from build123d import *


with BuildPart() as part:
    # Sketch1 → Revolve1 (revolve)
    with BuildSketch(Plane(origin=(0, 0, 0), x_dir=(0, 0, -1), z_dir=(1, 0, 0)), mode=Mode.PRIVATE) as revolve1_sk:
        with BuildLine():
            Line((-0.85, 1.95), (2.03, 1.95))
            Line((2.03, 1.95), (2.03, 1.5))
            Line((2.03, 1.5), (2.186173248, 1.2295))
            Line((2.186173248, 1.2295), (6.123826752, 1.2295))
            Line((6.123826752, 1.2295), (6.28, 1.5))
            Line((6.28, 1.5), (6.28, 2.100269256))
            Line((6.28, 2.100269256), (5.53, 2.45))
            Line((5.53, 2.45), (2.1, 2.45))
            ThreePointArc((2.1, 2.45), (1.94623106, 2.82123106), (1.575, 2.975))
            Line((1.575, 2.975), (1.02, 2.975))
            Line((1.02, 2.975), (1.02, 2.45))
            Line((1.02, 2.45), (0, 2.45))
            Line((0, 2.45), (0, 4))
            Line((0, 4), (-0.85, 4))
            Line((-0.85, 4), (-0.85, 1.95))
        make_face()
    revolve(revolve1_sk.sketch.rotate(Axis((0, 0, 0), (0, 0, -1)), 90), axis=Axis((0, 0, 0), (0, 0, -1)))


solid = part.part
Design review of the part built by this model. Coordinates are the model's own, in mm. A direction names the side the tool comes from. Coordinates: 2 decimals unless noted, no trailing zeros. Loops run counter-clockwise (first coordinate to the right, second up) from the corner with the lowest first, then second, coordinate; pieces in that order, holes last. Notation, with made-up numbers: (-36, 65) -> (-2, 65) arc R21 cw to (-2, 78) -> close; hole circle Ø3 at (41.5, 31). An arc over 180 degrees is marked (long way). Use a Markdown table: item, result. Add a question column.
Item 1: The part is to be moulded in two halves that separate along X. For faces 4 (the flat face through (2, -1, 0.85)), 5 (the cylindrical face through (-0.27, 1.2, -4.18)), 6 (the cylindrical face through (-2.2, -2, -1.3)), 7 (the cylindrical face through (-1.437, -1.318, -0.61)), say which applies: +X half, -X half, draft (parallel to the pull), parting line (faces both ways), or undercut.
Item 2: Clearance check with flat-ended pins moving along their axes: P1, Ø4, axis at x = 2, z = -2.5, coming from the -Y side; P2, Ø2, axis at y = 2.5, z = -5.5, coming from the -X side; P3, Ø4, axis at y = -2.5, z = -5.5, coming from the +X side. State where each tip first meets the part, or that it passes through.
Item 3: We need section C-C, the plane z = -5. Write out the cut boundary in (x, y), and give its area (3 significant figures).
Item 4: We need section D-D, the plane z = 0.25. Write out the cut boundary in (x, y), and give its area (3 significant figures).
Item 5: Wall thickness on L1, parallel to Y at x = 0, z = -0.5; L2, parallel to Z at x = 0, y = 2.5; L3, parallel to Y at x = 0, z = -3.8: over which ranges is each line inside the solid? List them lowest first. Write a range as from..to.
Item 6: Machinability: for faces 1 (the flat face through (-2, -2, 0)), 2 (the cylindrical face through (-0.867, 3.905, 0.431)), 3 (the cylindrical face through (-1.806, -1.656, -3.791)), which of the approach directions +Z, -Z, +X, -X, +Y, -Y give a long, thin tool a straight path to every point of the face, cutting with its end or side? Answer none if there is none.
Numbers:
| question | item | result |
|---|---|---|
| 1 | face 4 | draft |
| 1 | face 5 | undercut |
| 1 | face 6 | parting line |
| 1 | face 7 | undercut |
| 2 | P1 | stops at y = -2.97 |
| 2 | P2 | stops at x = -1.94 |
| 2 | P3 | stops at x = 2.4 |
| 3 | outline | circle Ø4.9 at (0, 0); hole circle Ø2.46 at (0, 0) |
| 3 | area | 14.1 mm^2 |
| 4 | outline | circle Ø8 at (0, 0); hole circle Ø3.9 at (0, 0) |
| 4 | area | 38.3 mm^2 |
| 5 | L1 | y = -2.45..-1.95, 1.95..2.45 |
| 5 | L2 | z = -2.1..-1.02, 0..0.85 |
| 5 | L3 | y = -2.45..-1.23, 1.23..2.45 |
| 6 | face 1 | none |
| 6 | face 2 | +Z, -Z |
| 6 | face 3 | -Z |
